```python
from build123d import *

# Parameters (mm, degrees)
SKETCH1_R           = 1.6
BOSS_EXTRUDE2_DEPTH = 3
FILLET1_R           = 3
CHAMFER1_SIZE       = 1.5


with BuildPart() as part:
    # Sketch1 → Boss-Extrude2 (new body)
    with BuildSketch(Plane(origin=(0, 0, 0), x_dir=(0, 0, -1), z_dir=(1, 0, 0))):
        with BuildLine():
            Line((0, 0), (105, 0))
            Line((105, 0), (105, 135))
            ThreePointArc((105, 135), (100.606601718, 145.606601718), (90, 150))
            Line((90, 150), (0, 150))
            Line((0, 150), (0, 0))
        make_face()
        with Locations((5, 145)):
            Circle(SKETCH1_R, mode=Mode.SUBTRACT)
        with Locations((97, 142)):
            Circle(SKETCH1_R, mode=Mode.SUBTRACT)
        with Locations((100, 5)):
            Circle(SKETCH1_R, mode=Mode.SUBTRACT)
        with Locations((5, 5)):
            Circle(SKETCH1_R, mode=Mode.SUBTRACT)
        Polygon((8.6, 145), (90, 145), (90, 135), (100, 135), (100, 8.6), align=None, mode=Mode.SUBTRACT)
        with BuildLine():
            Line((5, 10), (5, 141.4))
            Line((5, 141.4), (96.4, 5))
            Line((96.4, 5), (10, 5))
            ThreePointArc((10, 5), (8.535533906, 8.535533906), (5, 10))
        make_face(mode=Mode.SUBTRACT)
    extrude(amount=BOSS_EXTRUDE2_DEPTH)

    # Fillet1
    fillet1_edges = [part.edges().sort_by_distance(p)[0] for p in [
        (1.5, 5, -96.4),
        (1.5, 141.4, -5),
        (1.5, 145, -90),
        (1.5, 145, -8.6),
        (1.5, 8.6, -100),
        (1.5, 135, -100),
        (1.5, 135, -90),
    ]]
    fillet(fillet1_edges, radius=FILLET1_R)

    # Chamfer1
    chamfer1_edges = [part.edges().sort_by_distance(p)[0] for p in [
        (3, 5, -3.4),
        (3, 5, -98.4),
        (3, 142, -95.4),
        (3, 145, -3.4),
    ]]
    chamfer(chamfer1_edges, length=CHAMFER1_SIZE)


solid = part.part
```
Here's how the part is built. I have some questions about the finished solid (model axes, mm). A direction names the side the tool comes from. Round coordinates to 2 decimals unless told otherwise and drop trailing zeros. Order: outer loops, then holes, each group sorted by start corner. A loop starts at its lowest first (then second) coordinate and runs counter-clockwise, first axis right, second up. Notation, with made-up numbers: M 88.25,87 L 108.25,87 A32 cw 108.25,122 Z; hole C 37,-16 d10. An arc over 180 degrees is marked long. One line per question, with ' | ' between items.
1) For faces 1 (the face through (1, 67, -105)), 2 (the face through (1.479, 72.302, -51.302)), which set-ups out of +Z, -Z, +X, -X, +Y, -Y let a thin tool reach every point of the face, with its end or its side?
Working result:
face 1: -Z, +X, -X, +Y, -Y | face 2: +X, -X
2) I want a section at B-B, the plane y = 39. Write out the boundary of the cut face in (x, z).
Working result:
outline: M 0,-105 L 3,-105 L 3,-100 L 0,-100 Z; M 0,-79.63 L 3,-79.63 L 3,-73.62 L 0,-73.62 Z; M 0,-5 L 3,-5 L 3,0 L 0,0 Z
3) I need wall thicknesses on line 1 along Y through (x, z) = (1.9, -50.5); line 2 along Z through (x, y) = (0.1, 57); line 3 along Z through (x, y) = (1.3, 70). Which ranges of each line are inside material? Lowest first, please.
Working result:
line 1: 0 to 5, 73.5 to 82.47, 145 to 150 | line 2: -105 to -100, -67.57 to -61.56, -5 to 0 | line 3: -105 to -100, -58.86 to -52.84, -5 to 0
4) For pin 1 Ø2.5 at (y, z) = (145, -5) entering from +X, with a flat end and sliding along its axis, tell me the tip position at first contact or that it passes through.
Working result:
pin 1: through
5) If we mould it in two halves opening along Y, with no side actions, what happens to faces 3 (the face through (0.74, 3.44, -4.65)), 4 (the face through (3, 75, -52)), 5 (the face through (1, 0, -52)), 6 (the face through (1.48, 145.49, -100.72))? For each: +Y half, -Y half, draft (parallel to the pull), parting line (faces both ways), or undercut.
Working result:
face 3: undercut | face 4: draft | face 5: -Y half | face 6: +Y half
6) I want a section at A-A, the plane x = 2.15. Write out the boundary of the cut face in (y, z).
Working result:
outline: M 0,-105 L 135,-105 A15 ccw 150,-90 L 150,0 L 0,0 Z; hole C 5,-100 d4.5; hole C 5,-5 d4.5; hole M 5,-90.78 A3 ccw 9.67,-93.27 L 133.2,-10.49 A3 ccw 131.53,-5 L 10,-5 A5 cw 5,-10 Z; hole M 16.8,-94.51 A3 ccw 18.47,-100 L 132,-100 A3 ccw 135,-97 L 135,-93 A3 cw 138,-90 L 142,-90 A3 ccw 145,-87 L 145,-14.22 A3 ccw 140.33,-11.73 Z; hole C 142,-97 d4.5; hole C 145,-5 d4.5
7) I want a section at C-C, the plane z = -51. Write out the boundary of the cut face in (x, y).
Working result:
outline: M 0,0 L 3,0 L 3,5 L 0,5 Z; M 0,72.75 L 3,72.75 L 3,81.72 L 0,81.72 Z; M 0,145 L 3,145 L 3,150 L 0,150 Z
